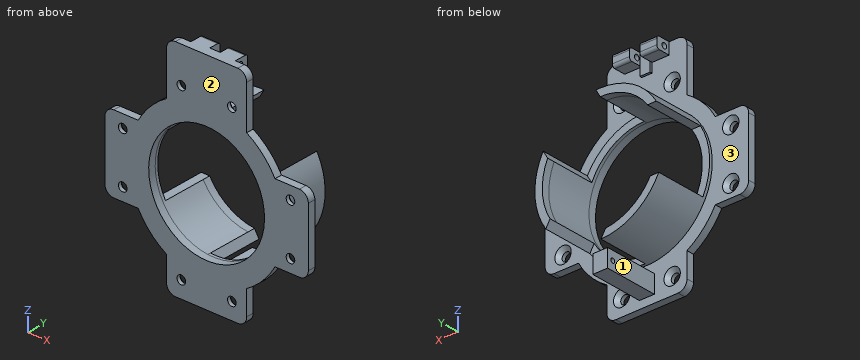
from build123d import *

# Parameters (mm, degrees)
BOSS_EXTRUDE3_DEPTH                          = 2.5
SKETCH1_6_R                                  = 22
SKETCH1_6_R_2                                = 19.5
BOSS_EXTRUDE4_DEPTH                          = 20.5
CUT_EXTRUDE2_REACH                           = 58.717
CUT_EXTRUDE2_END_RADIUS                      = 22
SKETCH33_W                                   = 21
SKETCH33_H                                   = 17
CIRPATTERN1_COUNT                            = 3
SKETCH1_7_R                                  = 19.5
CUT_EXTRUDE1_DEPTH                           = 18
CSK_FOR_M2_5_COUNTERSUNK_FLAT_HEAD_S_2_COUNT = 2
CSK_FOR_M2_5_COUNTERSUNK_FLAT_HEAD_S_2_PITCH = 17
CSK_FOR_M2_5_COUNTERSUNK_FLAT_HEAD_S_3_COUNT = 2
CSK_FOR_M2_5_COUNTERSUNK_FLAT_HEAD_S_3_PITCH = 41.706591715
CSK_FOR_M2_5_COUNTERSUNK_FLAT_HEAD_S_4_COUNT = 2
CSK_FOR_M2_5_COUNTERSUNK_FLAT_HEAD_S_4_PITCH = 51.957512596
CSK_FOR_M2_5_COUNTERSUNK_FLAT_HEAD_S_5_COUNT = 2
CSK_FOR_M2_5_COUNTERSUNK_FLAT_HEAD_S_5_PITCH = 58.982027644
CSK_FOR_M2_5_COUNTERSUNK_FLAT_HEAD_S_6_COUNT = 2
CSK_FOR_M2_5_COUNTERSUNK_FLAT_HEAD_S_6_PITCH = 56.47901898
CSK_FOR_M2_5_COUNTERSUNK_FLAT_HEAD_S_7_COUNT = 2
CSK_FOR_M2_5_COUNTERSUNK_FLAT_HEAD_S_7_PITCH = 27.915882035
CSK_FOR_M2_5_COUNTERSUNK_FLAT_HEAD_S_8_COUNT = 2
CSK_FOR_M2_5_COUNTERSUNK_FLAT_HEAD_S_8_PITCH = 41.706591715
SKETCH15_W                                   = 5.75
SKETCH15_H                                   = 3.91851851
SKETCH15_H_2                                 = 3.887074911
BOSS_EXTRUDE5_DEPTH                          = 4.75
SKETCH16_W                                   = 3.5
SKETCH16_H                                   = 7
BOSS_EXTRUDE6_DEPTH                          = 0.75
FILLET1_R                                    = 3
FILLET2_R                                    = 3
FILLET3_R                                    = 3
FILLET4_R                                    = 3
FILLET5_R                                    = 3
FILLET6_R                                    = 3
FILLET7_R                                    = 3
FILLET8_R                                    = 3
FILLET9_R                                    = 1
FILLET10_R                                   = 1
FILLET11_R                                   = 1
FILLET12_R                                   = 1
F_1_8_1_8_DIAMETER_HOLE2_D                   = 1.8
SKETCH22_W                                   = 5
SKETCH22_H                                   = 6
BOSS_EXTRUDE7_DEPTH                          = 18
F_1_5_1_5_DIAMETER_HOLE1_D                   = 1.5


with BuildPart() as part:
    # Sketch1 → Boss-Extrude3 (new body)
    with BuildSketch(Plane(origin=(0, 0, 0), x_dir=(1, 0, 0), z_dir=(0, 1, 0))):
        with BuildLine():
            Line((-34.253186733, 12.8), (-23.032205713, 12.8))
            ThreePointArc((-23.032205713, 12.8), (-18.915679134, 18.344470091), (-13.5, 22.62901898))
            Line((-13.5, 22.62901898), (-13.5, 33.85))
            Line((-13.5, 33.85), (13.5, 33.85))
            Line((13.5, 33.85), (13.5, 22.62901898))
            ThreePointArc((13.5, 22.62901898), (18.915679134, 18.344470091), (23.032205713, 12.8))
            Line((23.032205713, 12.8), (34.253186733, 12.8))
            Line((34.253186733, 12.8), (34.253186733, -12.8))
            Line((34.253186733, -12.8), (23.032205713, -12.8))
            ThreePointArc((23.032205713, -12.8), (18.915679134, -18.344470091), (13.5, -22.62901898))
            Line((13.5, -22.62901898), (13.5, -40.29))
            Line((13.5, -40.29), (-13.5, -40.29))
            Line((-13.5, -40.29), (-13.5, -22.62901898))
            ThreePointArc((-13.5, -22.62901898), (-18.915679134, -18.344470091), (-23.032205713, -12.8))
            Line((-23.032205713, -12.8), (-34.253186733, -12.8))
            Line((-34.253186733, -12.8), (-34.253186733, 12.8))
        make_face()
    extrude(amount=BOSS_EXTRUDE3_DEPTH)

    # Sketch1<6> → Boss-Extrude4 (add)
    with BuildSketch(Plane(origin=(0, 0, 0), x_dir=(1, 0, 0), z_dir=(0, 1, 0))):
        with Locations(Location((0, 0, 0), (0, 0, 270))):
            Circle(SKETCH1_6_R)
        with Locations(Location((0, 0, 0), (0, 0, 270))):
            Circle(SKETCH1_6_R_2, mode=Mode.SUBTRACT)
    extrude(amount=BOSS_EXTRUDE4_DEPTH)

    # Cut-Extrude2: up to this cylinder (the profile starts inside it)
    cut_extrude2_end = Plane(origin=(0, 12, 0), z_dir=(0, -1, 0)) * Cylinder(CUT_EXTRUDE2_END_RADIUS, 162.434, mode=Mode.PRIVATE)
    # Sketch33 → Cut-Extrude2 (cut, up to the surface)
    with BuildSketch(Plane(origin=(0, 0, 0), x_dir=(0, 0, -1), z_dir=(1, 0, 0)), mode=Mode.PRIVATE) as cut_extrude2_sk1:
        with Locations((-0.746304841, 12)):
            Rectangle(SKETCH33_W, SKETCH33_H)
    cut_extrude2_tool1 = extrude(cut_extrude2_sk1.sketch, amount=-CUT_EXTRUDE2_REACH, mode=Mode.PRIVATE) & cut_extrude2_end
    cut_extrude2 = cut_extrude2_tool1.solids().sort_by_distance((0, 12, 0.746305))[0]
    add(cut_extrude2, mode=Mode.SUBTRACT)

    # CirPattern1: Cut-Extrude2 ×3 about axis
    cirpattern1_axis = Axis((0, 0, 0), (0, 1, 0))
    for i in range(1, CIRPATTERN1_COUNT):
        add(cut_extrude2.rotate(cirpattern1_axis, i * 360 / CIRPATTERN1_COUNT), mode=Mode.SUBTRACT)

    # Sketch1<7> → Cut-Extrude1 (cut)
    with BuildSketch(Plane(origin=(0, 0, 0), x_dir=(1, 0, 0), z_dir=(0, 1, 0))):
        with Locations(Location((0, 0, 0), (0, 0, 95.221126585))):
            Circle(SKETCH1_7_R)
    extrude(amount=CUT_EXTRUDE1_DEPTH, mode=Mode.SUBTRACT)

    # Sketch14 → CSK for M2.5 Countersunk Flat Head Screw1 (revolve, cut)
    with BuildSketch(Plane(origin=(-8.5, 2.5, -28.23950949), x_dir=(0, 0, 1), z_dir=(1, 0, 0))):
        Polygon((0, 0), (0, 2.5), (1.45, 2.5), (1.45, 1.3), (2.75, 0), align=None)
    csk_for_m2_5_countersunk_flat_head_screw = revolve(axis=Axis((-8.5, 8.85, -28.23950949), (0, -1, 0)), mode=Mode.SUBTRACT)

    # CSK for M2.5 Countersunk Flat Head S 2: CSK for M2.5 Countersunk Flat Head Screw1 ×2
    with Locations(*[(i * CSK_FOR_M2_5_COUNTERSUNK_FLAT_HEAD_S_2_PITCH, 0, 0) for i in range(1, CSK_FOR_M2_5_COUNTERSUNK_FLAT_HEAD_S_2_COUNT)]):
        add(csk_for_m2_5_countersunk_flat_head_screw, mode=Mode.SUBTRACT)

    # CSK for M2.5 Countersunk Flat Head S 3: CSK for M2.5 Countersunk Flat Head Screw1 ×2
    with Locations(*[Vector(0.8809041443894198, 0, 0.4732947162155356) * (i * CSK_FOR_M2_5_COUNTERSUNK_FLAT_HEAD_S_3_PITCH) for i in range(1, CSK_FOR_M2_5_COUNTERSUNK_FLAT_HEAD_S_3_COUNT)]):
        add(csk_for_m2_5_countersunk_flat_head_screw, mode=Mode.SUBTRACT)

    # CSK for M2.5 Countersunk Flat Head S 4: CSK for M2.5 Countersunk Flat Head Screw1 ×2
    with Locations(*[Vector(0.7071067811865471, 0, 0.7071067811865479) * (i * CSK_FOR_M2_5_COUNTERSUNK_FLAT_HEAD_S_4_PITCH) for i in range(1, CSK_FOR_M2_5_COUNTERSUNK_FLAT_HEAD_S_4_COUNT)]):
        add(csk_for_m2_5_countersunk_flat_head_screw, mode=Mode.SUBTRACT)

    # CSK for M2.5 Countersunk Flat Head S 5: CSK for M2.5 Countersunk Flat Head Screw1 ×2
    with Locations(*[Vector(0.28822339073732456, 0, 0.9575631974088601) * (i * CSK_FOR_M2_5_COUNTERSUNK_FLAT_HEAD_S_5_PITCH) for i in range(1, CSK_FOR_M2_5_COUNTERSUNK_FLAT_HEAD_S_5_COUNT)]):
        add(csk_for_m2_5_countersunk_flat_head_screw, mode=Mode.SUBTRACT)

    # CSK for M2.5 Countersunk Flat Head S 6: CSK for M2.5 Countersunk Flat Head Screw1 ×2
    with Locations(*[(0, 0, i * CSK_FOR_M2_5_COUNTERSUNK_FLAT_HEAD_S_6_PITCH) for i in range(1, CSK_FOR_M2_5_COUNTERSUNK_FLAT_HEAD_S_6_COUNT)]):
        add(csk_for_m2_5_countersunk_flat_head_screw, mode=Mode.SUBTRACT)

    # CSK for M2.5 Countersunk Flat Head S 7: CSK for M2.5 Countersunk Flat Head Screw1 ×2
    with Locations(*[Vector(-0.7071067811865482, 0, 0.7071067811865469) * (i * CSK_FOR_M2_5_COUNTERSUNK_FLAT_HEAD_S_7_PITCH) for i in range(1, CSK_FOR_M2_5_COUNTERSUNK_FLAT_HEAD_S_7_COUNT)]):
        add(csk_for_m2_5_countersunk_flat_head_screw, mode=Mode.SUBTRACT)

    # CSK for M2.5 Countersunk Flat Head S 8: CSK for M2.5 Countersunk Flat Head Screw1 ×2
    with Locations(*[Vector(-0.4732947162155356, 0, 0.8809041443894198) * (i * CSK_FOR_M2_5_COUNTERSUNK_FLAT_HEAD_S_8_PITCH) for i in range(1, CSK_FOR_M2_5_COUNTERSUNK_FLAT_HEAD_S_8_COUNT)]):
        add(csk_for_m2_5_countersunk_flat_head_screw, mode=Mode.SUBTRACT)

    # Sketch15 → Boss-Extrude5 (add)
    with BuildSketch(Plane(origin=(0, 2.5, 0), x_dir=(1, 0, 0), z_dir=(0, 1, 0))):
        with Locations((4.625, -38.330740745)):
            Rectangle(SKETCH15_W, SKETCH15_H)
        with Locations((-4.625, -38.346462544)):
            Rectangle(SKETCH15_W, SKETCH15_H_2)
    extrude(amount=BOSS_EXTRUDE5_DEPTH)

    # Sketch16 → Boss-Extrude6 (add)
    with BuildSketch(Plane(origin=(0, 2.5, 0), x_dir=(1, 0, 0), z_dir=(0, 1, 0))):
        with Locations((0, -36.79)):
            Rectangle(SKETCH16_W, SKETCH16_H)
    extrude(amount=BOSS_EXTRUDE6_DEPTH)

    # Fillet1
    fillet1_edges = [part.edges().sort_by_distance(p)[0] for p in [
        (34.253186733, 1.25, 12.8),
    ]]
    fillet(fillet1_edges, radius=FILLET1_R)

    # Fillet2
    fillet2_edges = [part.edges().sort_by_distance(p)[0] for p in [
        (34.253186733, 1.25, -12.8),
    ]]
    fillet(fillet2_edges, radius=FILLET2_R)

    # Fillet3
    fillet3_edges = [part.edges().sort_by_distance(p)[0] for p in [
        (13.5, 1.25, -33.85),
    ]]
    fillet(fillet3_edges, radius=FILLET3_R)

    # Fillet4
    fillet4_edges = [part.edges().sort_by_distance(p)[0] for p in [
        (-13.5, 1.25, -33.85),
    ]]
    fillet(fillet4_edges, radius=FILLET4_R)

    # Fillet5
    fillet5_edges = [part.edges().sort_by_distance(p)[0] for p in [
        (-34.253186733, 1.25, -12.8),
    ]]
    fillet(fillet5_edges, radius=FILLET5_R)

    # Fillet6
    fillet6_edges = [part.edges().sort_by_distance(p)[0] for p in [
        (-34.253186733, 1.25, 12.8),
    ]]
    fillet(fillet6_edges, radius=FILLET6_R)

    # Fillet7
    fillet7_edges = [part.edges().sort_by_distance(p)[0] for p in [
        (-13.5, 1.25, 40.29),
    ]]
    fillet(fillet7_edges, radius=FILLET7_R)

    # Fillet8
    fillet8_edges = [part.edges().sort_by_distance(p)[0] for p in [
        (13.5, 1.25, 40.29),
    ]]
    fillet(fillet8_edges, radius=FILLET8_R)

    # Fillet9
    fillet9_edges = [part.edges().sort_by_distance(p)[0] for p in [
        (-4.625, 7.25, 36.402925089),
    ]]
    fillet(fillet9_edges, radius=FILLET9_R)

    # Fillet10
    fillet10_edges = [part.edges().sort_by_distance(p)[0] for p in [
        (-4.625, 7.25, 40.29),
    ]]
    fillet(fillet10_edges, radius=FILLET10_R)

    # Fillet11
    fillet11_edges = [part.edges().sort_by_distance(p)[0] for p in [
        (4.625, 7.25, 40.29),
    ]]
    fillet(fillet11_edges, radius=FILLET11_R)

    # Fillet12
    fillet12_edges = [part.edges().sort_by_distance(p)[0] for p in [
        (4.625, 7.25, 36.37148149),
    ]]
    fillet(fillet12_edges, radius=FILLET12_R)

    # Ø1.8 (1.8) Diameter Hole2 (through all)
    with Locations(Plane(origin=(7.5, 0, 0), x_dir=(0, 0, -1), z_dir=(1, 0, 0))):
        with Locations((-38.330740745, 4.4)):
            Hole(F_1_8_1_8_DIAMETER_HOLE2_D / 2)

    # Sketch22 → Boss-Extrude7 (add)
    with BuildSketch(Plane(origin=(0, 2.5, 0), x_dir=(1, 0, 0), z_dir=(0, 1, 0))):
        with Locations((0, 28.23950949)):
            Rectangle(SKETCH22_W, SKETCH22_H)
    extrude(amount=BOSS_EXTRUDE7_DEPTH)

    # Ø1.5 (1.5) Diameter Hole1 (through all)
    with Locations(Plane.ZY.offset(2.5)):
        with Locations((-28.23950949, 18.5)):
            Hole(F_1_5_1_5_DIAMETER_HOLE1_D / 2)


solid = part.part
Build history of the part. All positions in model axes, mm. Face numbers are marked on the shaded views. A direction names the side the tool comes from. Coordinates: 2 decimals unless noted, no trailing zeros. Order: outer loops, then holes, each group sorted by start corner. A loop starts at its lowest first (then second) coordinate and runs counter-clockwise, first axis right, second up. Notation, with made-up numbers: (19.25, 54) - (28.25, 54) arc R16 cw to (28.25, 85) - close; hole circle Ø6 at (-22.75, 31.5). An arc over 180 degrees is marked (long way). Write each question's results on one line, items separated by ' | '. Start each with the question number.
Item 1: Wall check: probe 1 along Z at (x, y) = (0, 13.75); probe 2 along X at (y, z) = (0.75, 8.5); probe 3 along Z at (x, y) = (-8.5, 0.55). Give the ranges that are in metal, low to high. Write a range as [from, to].
Item 2: Tool access for the marked faces 1, 2 and 3: list every direction of +Z, -Z, +X, -X, +Y, -Y with a clear straight run to the whole face (end or side of a thin tool).
Item 3: Band-saw the part on C-C on x = 15. Write the cut outline in (y, z), and give its area (3 significant figures).
Item 4: Band-saw the part on B-B on z = 0. Write the cut outline in (x, y).
Item 5: Band-saw the part on D-D on y = 4.4. State how many separate pieces and enclosed holes the cut face has, and give its area (3 significant figures).
Item 6: Flat gauge pins, fed straight in: pin 1 (3 mm diameter, centred on y = 4.5, z = 37.5, fed in from +X); pin 2 (0.6 mm diameter, centred on x = 5.5, z = 38.5, fed in from +Y); pin 3 (12 mm diameter, centred on y = 11.5, z = 9.5, fed in from +X); pin 4 (12 mm diameter, centred on x = 15, z = 17, fed in from -Y). Where does each tip first touch, or does it go through?
Item 7: Band-saw the part on A-A on y = 15.75. Write the cut outline in (x, z), and give its area (3 significant figures).
Numbers:
1) probe 1: [-31.24, -25.24], [19.51, 22] | probe 2: [-34.25, -29.69], [-26.79, -17.55], [17.55, 26.79], [29.69, 34.25] | probe 3: [-33.85, -29.69], [-26.79, -17.55], [17.55, 26.79], [29.69, 40.29]
2) face 1: -Z, -X, +Y | face 2: +Z, -Z, +X, -X, -Y | face 3: +Y
3) outline: (0, -21.66) - (2.5, -21.66) - (2.5, -16.09) - (3.5, -16.09) - (3.5, -12.46) - (0, -12.46) - close; (0, 12.46) - (3.5, 12.46) - (3.5, 16.09) - (2.5, 16.09) - (2.5, 21.66) - (0, 21.66) - close | area: 53.3 mm^2
4) outline: (-34.25, 0) - (-19.5, 0) - (-19.5, 3.5) - (-22, 3.5) - (-22, 2.5) - (-34.25, 2.5) - close; (19.5, 0) - (34.25, 0) - (34.25, 2.5) - (22, 2.5) - (22, 20.5) - (19.5, 20.5) - close
5) separate pieces: 8 | enclosed holes: 0 | area: 215 mm^2
6) pin 1: x = 7.5 | pin 2: y = 7.25 | pin 3: x = 21.72 | pin 4: y = 0
7) outline: (-19.72, -9.75) arc R22 ccw to (-0.29, -22) - (-1.77, -19.42) arc R19.5 cw to (-16.89, -9.75) - close; (-18.91, 11.25) - (-15.93, 11.25) arc R19.5 cw to (0, 19.5) - (1.41, 21.95) arc R22 ccw to start; (-2.5, -31.24) - (2.5, -31.24) - (2.5, -25.24) - (-2.5, -25.24) - close; (16.89, -9.75) - (18.31, -12.2) arc R22 ccw to (19.19, 10.75) - (17.7, 8.17) arc R19.5 cw to start | area: 191 mm^2
